Part print with two shaded views. Sizes in mm from the minimum x, y, z corner. Coordinates: 2 decimals unless noted, no trailing zeros. Loops run counter-clockwise (first coordinate to the right, second up) from the corner with the lowest first, then second, coordinate; pieces in that order, holes last.
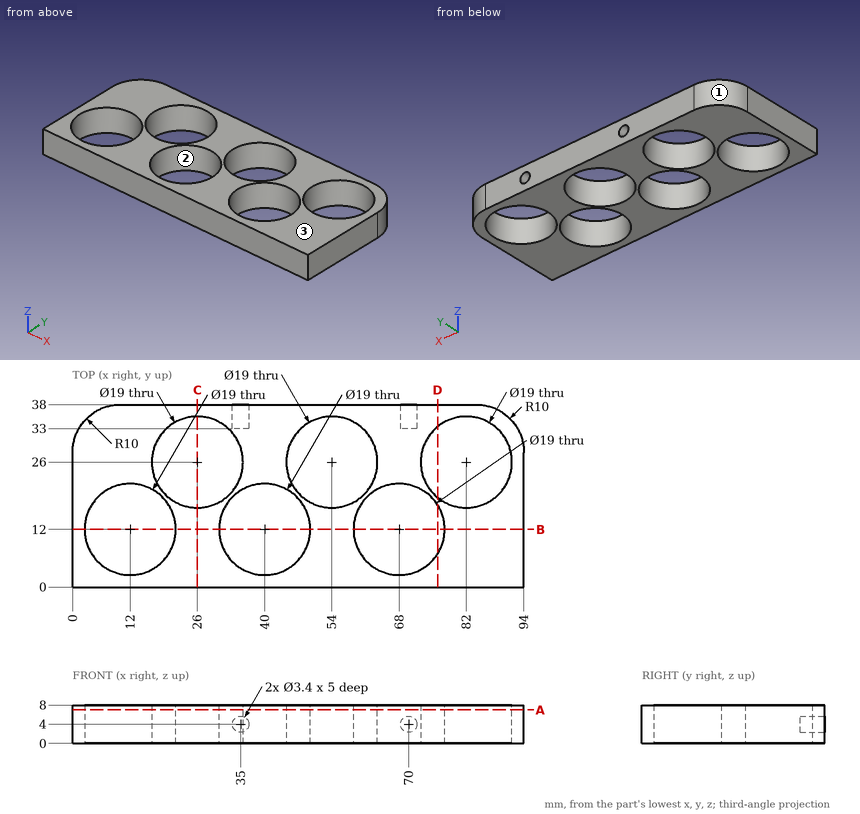
Q1. Slice it at D-D (x = 76). List the corners of the cut face in (y, z), and give its area (3 significant figures).
Answers:
outline: (0, 0) - (6.88, 0) - (6.88, 8) - (0, 8) - close; (17.12, 0) - (18.63, 0) - (18.63, 8) - (17.12, 8) - close; (33.37, 0) - (38, 0) - (38, 8) - (33.37, 8) - close
area: 104 mm2
Q2. Slice it at C-C (x = 26). List the corners of the cut face in (y, z).
Answers:
outline: (0, 0) - (16.5, 0) - (16.5, 8) - (0, 8) - close; (35.5, 0) - (38, 0) - (38, 8) - (35.5, 8) - close
Q3. Slice it at B-B (y = 12). List the corners of the cut face in (x, z), and give its area (3 significant figures).
Answers:
outline: (0, 0) - (2.5, 0) - (2.5, 8) - (0, 8) - close; (21.5, 0) - (30.5, 0) - (30.5, 8) - (21.5, 8) - close; (49.5, 0) - (58.5, 0) - (58.5, 8) - (49.5, 8) - close; (77.5, 0) - (94, 0) - (94, 8) - (77.5, 8) - close
area: 296 mm2
Q4. Flat gauge pins, fed straight in: P1, Ø3, axis at x = 84, y = 10, coming from the -Z side; P2, Ø2.5, axis at x = 70, z = 4, coming from the +Y side. Where does each tip first touch, or does it go through?
Answers:
P1: stops at z = 0
P2: stops at y = 33
Q5. Drill centre lines: line 1 (X direction, y = 3.5, z = 6); line 2 (X direction, y = 36.05, z = 4); line 3 (Y direction, x = 54, z = 4.25). Where is each one in solid material? Low to high.
Answers:
line 1: x = 0 to 7.76, 16.24 to 35.76, 44.24 to 63.76, 72.24 to 94
line 2: x = 4.07 to 33.3, 36.7 to 68.3, 71.7 to 89.93
line 3: y = 0 to 16.5, 35.5 to 38
Q6. Slice it at A-A (z = 7). List the corners of the cut face in (x, y).
Answers:
outline: (0, 0) - (94, 0) - (94, 28) arc R10 ccw to (84, 38) - (10, 38) arc R10 ccw to (0, 28) - close; hole circle Ø19 at (12, 12); hole circle Ø19 at (26, 26); hole circle Ø19 at (40, 12); hole circle Ø19 at (54, 26); hole circle Ø19 at (68, 12); hole circle Ø19 at (82, 26)
Q7. Mould opens along Y. For the marked faces 1, 2 and 3 say: +Y half, -Y half, draft (parallel to the pull), parting line (faces both ways), or undercut.
Answers:
face 1: +Y half
face 2: undercut
face 3: draft
